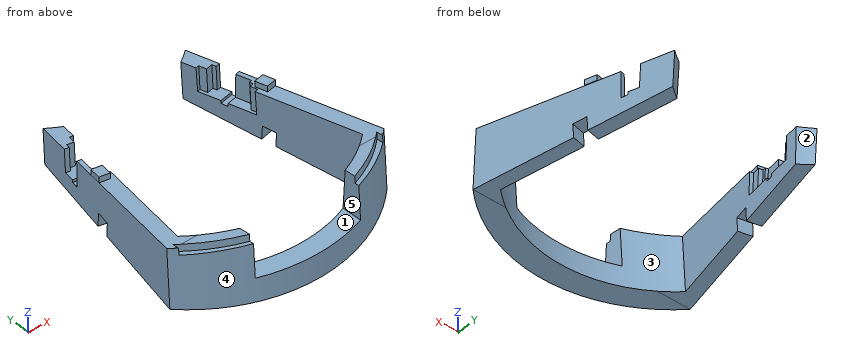
from build123d import *

# Parameters (mm, degrees)
BOSS_EXTRUDE1_DEPTH     = 209.55
SKETCH3_W               = 240.510539239
SKETCH3_H               = 265.315522901
CUT_EXTRUDE1_DEPTH      = 61.780833862
CUT_EXTRUDE2_DEPTH      = 59.88645018
CUT_EXTRUDE3_DEPTH      = 12.7
CUT_EXTRUDE4_DEPTH      = 6.35
SKETCH7_W               = 101.6
SKETCH7_H               = 37.465
CUT_EXTRUDE5_DEPTH      = 178.176697197
CUT_EXTRUDE5_DEPTH_BACK = 42.974613266
SKETCH10_R              = 2.667
CUT_EXTRUDE8_DEPTH      = 50.8
SKETCH11_R              = 2.667
CUT_EXTRUDE9_DEPTH      = 50.8
BOSS_EXTRUDE2_DEPTH     = 5.08
CUT_EXTRUDE10_DEPTH     = 19.05
CUT_EXTRUDE11_DEPTH     = 19.05
CUT_EXTRUDE12_DEPTH     = 20.955


with BuildPart() as part:
    # Sketch2 → Boss-Extrude1 (new body)
    with BuildSketch(Plane(origin=(0, 0, 0), x_dir=(0, 0, -1), z_dir=(1, 0, 0))):
        Polygon((-42.945985173, 177.447146824), (-53.974998987, -0.010456153), (-57.520039142, -57.050399967), (3.378068797, -53.539609111), (0, 0), (-11.195985173, 177.447146824), align=None)
    extrude(amount=BOSS_EXTRUDE1_DEPTH)

    # Sketch3 → Cut-Extrude1 (cut, through all)
    with BuildSketch(Plane(origin=(0, 3.341605618, 53.766667899), x_dir=(1, 0, 0), z_dir=(0, 0.062030449, 0.998074257))):
        with Locations((107.411926899, 58.645471754)):
            Rectangle(SKETCH3_W, SKETCH3_H)
        with BuildLine():
            Line((172.901684058, 173.982013262), (209.55, 0))
            ThreePointArc((209.55, 0), (104.775, -41.729500882), (0, 0))
            Line((0, 0), (35.741813567, 174.170499118))
            ThreePointArc((35.741813567, 174.170499118), (104.287966167, 149.492856038), (172.901684058, 173.982013262))
        make_face(mode=Mode.SUBTRACT)
    extrude(amount=-CUT_EXTRUDE1_DEPTH, mode=Mode.SUBTRACT)

    # Sketch4 → Cut-Extrude2 (cut, through all)
    with BuildSketch(Plane(origin=(0, 0, 0), x_dir=(-1, 0, 0), z_dir=(0, 0.062969545, -0.998015449))):
        with BuildLine():
            Line((-160.868955232, 170.846287594), (-193.979445404, 12.421844718))
            ThreePointArc((-193.979445404, 12.421844718), (-104.775, -21.808079515), (-15.570554596, 12.421844718))
            Line((-15.570554596, 12.421844718), (-48.003667802, 170.846287594))
            Line((-48.003667802, 170.846287594), (-160.868955232, 170.846287594))
        make_face()
    extrude(amount=-CUT_EXTRUDE2_DEPTH, mode=Mode.SUBTRACT)

    # Sketch5 → Cut-Extrude3 (cut)
    with BuildSketch(Plane(origin=(0, 0, 0), x_dir=(-1, 0, 0), z_dir=(0, 0.062969545, -0.998015449))):
        Polygon((-189.575592117, 100.998599654), (-176.057501646, 98.17333738), (-178.65564658, 85.741939916), (-192.173737051, 88.56720219), align=None)
        Polygon((-33.125849843, 98.17333738), (-19.492211444, 100.964455529), (-16.94721956, 88.533058065), (-30.58085796, 85.741939916), align=None)
    extrude(amount=-CUT_EXTRUDE3_DEPTH, mode=Mode.SUBTRACT)

    # Sketch6 → Cut-Extrude4 (cut)
    with BuildSketch(Plane(origin=(0, 3.341605618, 53.766667899), x_dir=(1, 0, 0), z_dir=(0, 0.062030449, 0.998074257))):
        with BuildLine():
            Line((6.35, -5.683612864), (6.35, 0.666387136))
            ThreePointArc((6.35, 0.666387136), (104.775, -38.257263578), (203.2, 0.666387136))
            Line((203.2, 0.666387136), (203.2, -5.683612864))
            ThreePointArc((203.2, -5.683612864), (104.775, -41.729500882), (6.35, -5.683612864))
        make_face()
    extrude(amount=-CUT_EXTRUDE4_DEPTH, mode=Mode.SUBTRACT)

    # Sketch7 → Cut-Extrude5 (cut, two sides)
    with BuildSketch(Plane(origin=(0, 0, 0), x_dir=(1, 0, 0), z_dir=(0, 1, 0))) as cut_extrude5_sk:
        with Locations((104.775, -37.622667571)):
            Rectangle(SKETCH7_W, SKETCH7_H)
    extrude(amount=CUT_EXTRUDE5_DEPTH, mode=Mode.SUBTRACT)
    extrude(cut_extrude5_sk.sketch, amount=-CUT_EXTRUDE5_DEPTH_BACK, mode=Mode.SUBTRACT)

    # Sketch10 → Cut-Extrude8 (cut)
    with BuildSketch(Plane(origin=(200.647085604, 42.183769093, -2.621726904), x_dir=(-0.012512246, -0.002630558, -0.999918259), z_dir=(0.978526509, 0.205724076, -0.012785779))):
        with Locations(Location((-34.774476568, 102.235809265, 0), (0, 0, 90))):  # turned: the seam where the file's is
            Circle(SKETCH10_R)
    extrude(amount=-CUT_EXTRUDE8_DEPTH, mode=Mode.SUBTRACT)

    # Sketch11 → Cut-Extrude9 (cut)
    with BuildSketch(Plane(origin=(0, 0, 0), x_dir=(-0.012215925, 0.002502022, 0.999922253), z_dir=(-0.979586609, 0.200635456, -0.01246952))):
        with Locations(Location((32.158429543, 145.097393201, 0), (0, 0, 270))):  # turned: the seam where the file's is
            Circle(SKETCH11_R)
    extrude(amount=-CUT_EXTRUDE9_DEPTH, mode=Mode.SUBTRACT)

    # Sketch13 → Boss-Extrude2 (add)
    with BuildSketch(Plane(origin=(0, 3.341605618, 53.766667899), x_dir=(1, 0, 0), z_dir=(0, 0.062030449, 0.998074257))):
        Polygon((21.844, 106.446204126), (19.546311985, 95.249529182), (29.001281937, 93.309259303), (31.298969952, 104.505934246), align=None)
        Polygon((178.251030048, 104.505934246), (187.706, 106.446204126), (190.003688015, 95.249529182), (180.548718063, 93.309259303), align=None)
    extrude(amount=BOSS_EXTRUDE2_DEPTH)

    # Sketch14 → Cut-Extrude10 (cut)
    with BuildSketch(Plane(origin=(0, 0, 0), x_dir=(-0.012215925, 0.002502022, 0.999922253), z_dir=(-0.979586609, 0.200635456, -0.01246952))):
        Polygon((45.523011798, 138.747393201), (45.909608937, 132.397393201), (22.028011798, 132.397393201), (22.028011798, 138.747393201), align=None)
    extrude(amount=-CUT_EXTRUDE10_DEPTH, mode=Mode.SUBTRACT)

    # Sketch15 → Cut-Extrude11 (cut)
    with BuildSketch(Plane(origin=(200.647085604, 42.183769093, -2.621726904), x_dir=(-0.012512246, -0.002630558, -0.999918259), z_dir=(0.978526509, 0.205724076, -0.012785779))):
        Polygon((-48.138588614, 95.885809265), (-24.643588614, 95.885809265), (-24.643588614, 89.535809265), (-48.52476738, 89.535809265), align=None)
    extrude(amount=-CUT_EXTRUDE11_DEPTH, mode=Mode.SUBTRACT)

    # Sketch16 → Cut-Extrude12 (cut)
    with BuildSketch(Plane(origin=(0, 3.341605618, 53.766667899), x_dir=(1, 0, 0), z_dir=(0, 0.062030449, 0.998074257))):
        Polygon((45.273381068, 151.976469085), (41.976582335, 152.653010556), (40.572439659, 145.81059809), (34.352064691, 147.087091432), (33.586168686, 143.354866451), (29.586519575, 144.175641), (27.283705248, 132.953985446), (31.283354359, 132.133210897), (27.13987731, 111.94197286), (29.628027298, 111.431375523), (28.988403038, 108.314475026), (32.720628019, 107.548579021), (31.316485344, 100.706166555), (34.718800408, 100.015076365), align=None)
        Polygon((174.153822626, 100.015076365), (163.599241965, 151.976469085), (166.896040699, 152.653010556), (168.300183374, 145.81059809), (174.520558343, 147.087091432), (175.286454348, 143.354866451), (179.286103459, 144.175641), (181.588917786, 132.953985446), (177.589268675, 132.133210897), (181.732745723, 111.94197286), (179.244595736, 111.431375523), (179.884219995, 108.314475026), (176.151995014, 107.548579021), (177.55613769, 100.706166555), align=None)
    extrude(amount=-CUT_EXTRUDE12_DEPTH, mode=Mode.SUBTRACT)


solid = part.part
Read the model definition and answer for the solid it produces. Units are mm, in the model's axes. Face numbers are marked on the shaded views. A direction names the side the tool comes from. Round coordinates to 2 decimals unless told otherwise and drop trailing zeros. Order: outer loops, then holes, each group sorted by start corner. A loop starts at its lowest first (then second) coordinate and runs counter-clockwise, first axis right, second up.
1) The mould has two halves that part along Y. Classify the marked faces 3, 4 and 5: released by +Y, released by -Y, zero draft, split by the parting line, or undercut.
2) The part is cut by section A-A on y = 31.5. Write down the section's boundary in (x, z), plus the area to 3 significant figures.
3) Flat-ended cylindrical pins translate along their axes: pin 1 (15 mm diameter, centred on y = -20, z = 29, fed in from -X); pin 2 (5.5 mm diameter, centred on y = 1.5, z = 50.5, fed in from +X); pin 3 (5 mm diameter, centred on y = -10, z = 17, fed in from +X); pin 4 (7.5 mm diameter, centred on y = 0, z = 51, fed in from -X). Find the tip coordinate at first contact, or state that the pin passes through.
4) The part is cut by section B-B on z = 37. Give the number of separate pieces and of enclosed holes in the cut face, plus the area to 3 significant figures.
5) Straight lines are drawn through the part: L1, parallel to X at y = 18, z = 19; L2, parallel to X at y = 22.5, z = 44; L3, parallel to Z at x = 23, y = 103.5. For each, find the intervals that lie inside material, in ascending order.
6) The part is cut by section C-C on y = 122. Write down the section's boundary in (x, z).
7) For the marked faces 1 and 2, determine the directions among +Z, -Z, +X, -X, +Y, -Y from which every point of the face is accessible in a straight line to the end or side of a thin tool.
8) The part is cut by section D-D on x = 82. Write down the section's boundary in (y, z).
Resolved:
1. face 3: undercut
1. face 4: released by -Y
1. face 5: zero draft
2. outline: (5.79, 52.02) - (6.43, 1.99) - (19.49, 1.99) - (20.13, 52.02) - close; (189.32, 52.02) - (189.98, 1.99) - (202.95, 1.99) - (203.61, 52.02) - close
2. area: 1,370 mm2
3. pin 1: stops at x = 17.49
3. pin 2: stops at x = 209.55
3. pin 3: stops at x = 199.73
3. pin 4: stops at x = 0
4. separate pieces: 4
4. enclosed holes: 0
4. area: 5,390 mm2
5. L1: x = 3.44 to 16.95, 192.57 to 206.01
5. L2: x = 4.05 to 18.19, 191.3 to 205.39
5. L3: z = 6.53 to 52.63
6. outline: (24.4, 46.39) - (24.89, 7.7) - (38.05, 7.7) - (38.28, 25.4) - (28.83, 25.4) - (28.57, 46.39) - close; (170.79, 25.4) - (171.03, 7.7) - (184, 7.7) - (184.51, 46.39) - (180.31, 46.39) - (180.04, 25.4) - close
7. face 1: +Z, +Y, -Y
7. face 2: -Z, +Y
8. outline: (-40.25, -2.54) - (-19.81, -1.25) - (-21.08, 18.89) - (-38.92, 18.89) - close
